from build123d import *

# Parameters (mm, degrees)
CROQUIS1_R                     = 3
CROQUIS1_R_2                   = 4
CROQUIS1_R_3                   = 5
SALIENTE_EXTRUIR1_DEPTH        = 25
CHAFL_N1_SIZE                  = 1
CORTAR_EXTRUIR1_DEPTH          = 94.3
CROQUIS3_R                     = 4.25
CORTAR_EXTRUIR2_DEPTH          = 94.3
CROQUIS4_R                     = 6.5
CORTAR_EXTRUIR3_DEPTH          = 8
CROQUIS5_R                     = 12.5
CORTAR_EXTRUIR4_DEPTH          = 141.5
TALADRO_ROSCADO_M10X1_01_D     = 9
TALADRO_ROSCADO_M10X1_01_DEPTH = 20
TALADRO_ROSCADO_M10X1_01_TIP   = 2.703872786


with BuildPart() as part:
    # Croquis1 → Saliente-Extruir1 (new body, symmetric)
    with BuildSketch(Plane.XY):
        Polygon((0, 0), (125, 0), (125, -62), (117, -70), (30, -70), (0, -40), align=None)
        with Locations((10, -15)):
            Circle(CROQUIS1_R, mode=Mode.SUBTRACT)
        with Locations((10, -35.8)):
            Circle(CROQUIS1_R_2, mode=Mode.SUBTRACT)
        with Locations((45, -35.8)):
            Circle(CROQUIS1_R_3, mode=Mode.SUBTRACT)
        with Locations((98.6, -57.2)):
            Circle(CROQUIS1_R_3, mode=Mode.SUBTRACT)
    extrude(amount=SALIENTE_EXTRUIR1_DEPTH, both=True)

    # Chaflán1
    chafl_n1_edges = [part.edges().sort_by_distance(p)[0] for p in [
        (0, 0, 0),
        (125, 0, 0),
        (62.5, 0, 25),
        (62.5, 0, -25),
    ]]
    chamfer(chafl_n1_edges, length=CHAFL_N1_SIZE)

    # Croquis2 → Cortar-Extruir1 (cut)
    with BuildSketch(Plane(origin=(0, 0, 0), x_dir=(1, 0, 0), z_dir=(0, 1, 0))):
        with BuildLine():
            Line((30, 2), (-5.316293701, 2))
            Line((-5.316293701, 2), (-5.316293701, -2))
            Line((-5.316293701, -2), (30, -2))
            ThreePointArc((30, -2), (32, 0), (30, 2))
        make_face()
    extrude(amount=-CORTAR_EXTRUIR1_DEPTH, mode=Mode.SUBTRACT)

    # Croquis3 → Cortar-Extruir2 (cut)
    with BuildSketch(Plane(origin=(0, 0, 2), x_dir=(-1, 0, 0), z_dir=(0, 0, -1))):
        with Locations((-10, -35.8)):
            Circle(CROQUIS3_R)
    extrude(amount=-CORTAR_EXTRUIR2_DEPTH, mode=Mode.SUBTRACT)

    # Croquis4 → Cortar-Extruir3 (cut)
    with BuildSketch(Plane.XY.offset(25)):
        with Locations((10, -35.8)):
            Circle(CROQUIS4_R)
    extrude(amount=-CORTAR_EXTRUIR3_DEPTH, mode=Mode.SUBTRACT)

    # Croquis5 → Cortar-Extruir4 (cut)
    with BuildSketch(Plane(origin=(125, 0, 0), x_dir=(0, 0, -1), z_dir=(1, 0, 0))):
        with Locations((0, -15)):
            Circle(CROQUIS5_R)
    extrude(amount=-CORTAR_EXTRUIR4_DEPTH, mode=Mode.SUBTRACT)

    # Taladro roscado M10x1.01
    with Locations(Plane(origin=(125, 0, 0), x_dir=(0, 0, -1), z_dir=(1, 0, 0))):
        with Locations((0, -45)):
            Hole(TALADRO_ROSCADO_M10X1_01_D / 2, depth=TALADRO_ROSCADO_M10X1_01_DEPTH)
            with Locations((0, 0, -(TALADRO_ROSCADO_M10X1_01_DEPTH + TALADRO_ROSCADO_M10X1_01_TIP / 2))):  # 118° drill point
                Cone(0, TALADRO_ROSCADO_M10X1_01_D / 2, TALADRO_ROSCADO_M10X1_01_TIP, mode=Mode.SUBTRACT)


solid = part.part
The listing builds one solid part. Answer for the finished solid, in the listing's coordinates (mm). A direction names the side the tool comes from. Coordinates: 2 decimals unless noted, no trailing zeros. Write each loop counter-clockwise with the first axis right and the second up, starting at its lowest first coordinate (ties: lowest second). Pieces come first, ordered by that corner, then holes. Notation, with made-up numbers: (59.25, 78.25) - (100.25, 78.25) arc R19 cw to (100.25, 94.25) - close; hole circle Ø10 at (30.5, -9). An arc over 180 degrees is marked (long way). Answer as CSV lines item,"result".
1. Straight lines are drawn through the part: line 1 (X direction, y = -35.5, z = -12); line 2 (Z direction, x = 66, y = -15); line 3 (X direction, y = -15, z = -17). For each, find the intervals that lie inside material, in ascending order. Write a range as [from, to].
Computed values:
line 1,"x = [0, 6.01], [13.99, 40.01], [49.99, 125]"
line 2,"z = [-25, -12.5], [12.5, 25]"
line 3,"x = [0, 7], [13, 125]"
2. Find section B-B (y = -15). Give the vertices of the cut face in (x, z), plus the area to 4 significant figures.
Computed values:
outline,"(0, -25) - (7, -25) - (7, -12.5) - (0, -12.5) - close; (0, 12.5) - (7, 12.5) - (7, 25) - (0, 25) - close; (13, -25) - (125, -25) - (125, -12.5) - (13, -12.5) - close; (13, 12.5) - (125, 12.5) - (125, 25) - (13, 25) - close"
area,"2,975 mm²"
3. Find section A-A (x = 22.5). Give the vertices of the cut face in (y, z).
Computed values:
outline,"(-62.5, -25) - (-1, -25) - (0, -24) - (0, -2) - (-2.66, -2) arc R12.5 cw to (-27.34, -2) - (-62.5, -2) - close; (-62.5, 2) - (-27.34, 2) arc R12.5 cw to (-2.66, 2) - (0, 2) - (0, 24) - (-1, 25) - (-62.5, 25) - close"
4. Given P1, Ø3, axis at y = -24, z = 5.5, coming from the -X side; P2, Ø4, axis at x = 7.5, y = -36, coming from the +Z side; P3, Ø10, axis at x = 21, z = -13, coming from the -Y side, each flat-ended and moving along its own axis, determine where each tip first touches the part or whether it passes through.
Computed values:
P1,"passes through"
P2,"stops at z = 17"
P3,"stops at y = -66"
5. Determine the mould class of faces 6 (the flat face through (18, -44, 2)), 7 (the flat face through (15, -55, -13)), 8 (the cylindrical face through (6.8, -38.2, -13.7)), 9 (the cylindrical face through (97.949, -52.243, -0.35)) for opening direction Y: +Y half, -Y half, draft (parallel to the pull), parting line (faces both ways), or undercut.
Computed values:
face 6,"draft"
face 7,"-Y half"
face 8,"undercut"
face 9,"undercut"
6. Find section D-D (z = 21.5). Give the vertices of the cut face in (x, y).
Computed values:
outline,"(0, -40) - (30, -70) - (117, -70) - (125, -62) - (125, -1) - (124, 0) - (1, 0) - (0, -1) - close; hole circle Ø13 at (10, -35.8); hole circle Ø6 at (10, -15); hole circle Ø10 at (45, -35.8); hole circle Ø10 at (98.6, -57.2)"
7. A tool of negligible diameter and unlimited length cuts with its end or side. For faces 1 (the cylindrical face through (114.86, -49.39, -0.98)), 2 (the flat face through (19, -44, -2)), 3 (the flat face through (62, 0, 0)), 4 (the flat face through (11.4, -40, 17)), 5 (the flat face through (74, -70, 0)), from which of +Z, -Z, +X, -X, +Y, -Y can it reach the whole face along a straight path? Write none if from no direction.
Computed values:
face 1,"+X"
face 2,"-X, +Y, -Y"
face 3,"+Z, -Z, +X, -X, +Y"
face 4,"+Z"
face 5,"+Z, -Z, +X, -X, -Y"
8. Find section C-C (y = -57.2). Give the vertices of the cut face in (x, z).
Computed values:
outline,"(17.2, -25) - (93.6, -25) - (93.6, 25) - (17.2, 25) - (17.2, 2) - (30, 2) arc R2 cw to (30, -2) - (17.2, -2) - close; (103.6, -25) - (125, -25) - (125, 25) - (103.6, 25) - close"
